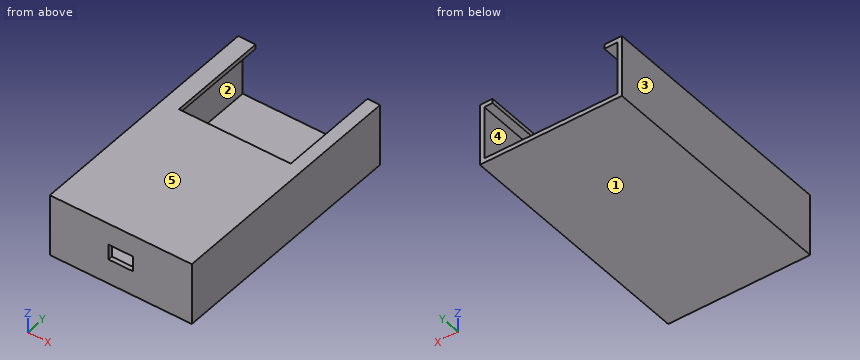
from build123d import *

# Parameters (mm, degrees)
F0_W     = 80
F0_H     = 140
F1_DEPTH = 35
F2_T     = -2.5
F3_W     = 63
F3_H     = 57
F4_DEPTH = 2.5
F5_W     = 13.924362
F5_H     = 8.664047
F6_DEPTH = 140.001


with BuildPart() as f1:
    # F0 (on Top) → F1 (new body)
    with BuildSketch(Plane.XY):
        Rectangle(F0_W, F0_H)
    extrude(amount=F1_DEPTH)

    # F2
    f2_openings = [f1.faces().sort_by_distance(p)[0] for p in [
        (0, 70, 17.5),
    ]]
    offset(amount=F2_T, openings=f2_openings)

    # F3 (on face) → F4 (cut)
    with BuildSketch(Plane.XY.offset(35)):
        with Locations((1.330548, 41.5)):
            Rectangle(F3_W, F3_H)
    extrude(amount=-F4_DEPTH, mode=Mode.SUBTRACT)

    # F5 (on face) → F6 (cut, through all)
    with BuildSketch(Plane.XZ.offset(70)):
        with Locations((0, 18.42829)):
            Rectangle(F5_W, F5_H)
    extrude(amount=-F6_DEPTH, mode=Mode.SUBTRACT)


solid = f1.part
Work out the finished part from the listing and answer in its coordinate system (mm). Face numbers are marked on the shaded views. A direction names the side the tool comes from. Round coordinates to 2 decimals unless told otherwise and drop trailing zeros. Loops run counter-clockwise (first coordinate to the right, second up) from the corner with the lowest first, then second, coordinate; pieces in that order, holes last. Notation, with made-up numbers: (74.25, 23) -> (129.25, 23) arc R19 ccw to (129.25, 46) -> close; hole circle Ø9 at (-0.5, 24.25). An arc over 180 degrees is marked (long way). Use one line per item in the form item = value.
(1) Find section D-D on y = 55.5. Give the vertices of the cut face in (x, z).
Answer list:
outline = (-40, 0) -> (40, 0) -> (40, 35) -> (32.83, 35) -> (32.83, 32.5) -> (37.5, 32.5) -> (37.5, 2.5) -> (-37.5, 2.5) -> (-37.5, 32.5) -> (-30.17, 32.5) -> (-30.17, 35) -> (-40, 35) -> close
(2) Straight lines are drawn through the part: line 1 (Z direction, x = -28, y = -16.5); line 2 (X direction, y = -56, z = 10.5); line 3 (Z direction, x = -8, y = 34.5). For each, find the intervals that lie inside material, in ascending order.
Answer list:
line_1 = 0 to 2.5, 32.5 to 35
line_2 = -40 to -37.5, 37.5 to 40
line_3 = 0 to 2.5
(3) Find section A-A on y = -34. Give the vertices of the cut face in (x, z), then the cut area to 3 significant figures.
Answer list:
outline = (-40, 0) -> (40, 0) -> (40, 35) -> (-40, 35) -> close; hole (-37.5, 2.5) -> (37.5, 2.5) -> (37.5, 32.5) -> (-37.5, 32.5) -> close
area = 550 mm2
(4) Flat-ended cylindrical pins translate along their axes: P1, Ø4, axis at x = 24.5, z = 8, coming from the +Y side; P2, Ø1.2, axis at x = -8, z = 33.5, coming from the +Y side. Find the tip coordinate at first contact, or state that the pin passes through.
Answer list:
P1 = -67.5
P2 = 13
(5) Find section B-B on x = 3. Give the vertices of the cut face in (y, z).
Answer list:
outline = (-70, 0) -> (70, 0) -> (70, 2.5) -> (-67.5, 2.5) -> (-67.5, 14.1) -> (-70, 14.1) -> close; (-70, 22.76) -> (-67.5, 22.76) -> (-67.5, 32.5) -> (13, 32.5) -> (13, 35) -> (-70, 35) -> close
(6) Find section C-C on z = 7. Give the vertices of the cut face in (x, y), then the cut area to 4 significant figures.
Answer list:
outline = (-40, -70) -> (40, -70) -> (40, 70) -> (37.5, 70) -> (37.5, -67.5) -> (-37.5, -67.5) -> (-37.5, 70) -> (-40, 70) -> close
area = 887.5 mm2
(7) For a pull along Z with two mould halves and no side action, classify the marked faces 3, 4 and 5 as released by +Z, released by -Z, zero draft, split by the parting line, or undercut.
Answer list:
face_3 = zero draft
face_4 = undercut
face_5 = released by +Z
(8) A tool of negligible diameter and unlimited length cuts with its end or side. For the marked faces 1 and 2, from which of +Z, -Z, +X, -X, +Y, -Y can it reach the whole face along a straight path? Write none if from no direction.
Answer list:
face_1 = -Z, +X, -X, +Y, -Y
face_2 = +Y
